Source: CAD feature listing. Evaluate the final solid. Frame: model axes, mm. A direction names the side the tool comes from. Give positions to 0.01 mm unless a question says otherwise; leave off trailing zeros. Write each loop counter-clockwise with the first axis right and the second up, starting at its lowest first coordinate (ties: lowest second). Pieces come first, ordered by that corner, then holes. Notation, with made-up numbers: (68, -11.75) -> (112, -11.75) arc R20 cw to (112, 15.25) -> close; hole circle Ø4 at (-7, 63). An arc over 180 degrees is marked (long way). Write item = value, one per line.
from build123d import *

# Parameters (mm, degrees)
F0_W     = 6.35
F0_H     = 2.54
F1_DEPTH = 19.05
F2_W     = 6.35
F2_H     = 5.588
F3_DEPTH = 2.54
F4_R     = 1.5875
F5_DEPTH = 25.4


with BuildPart() as f1:
    # F0 (on Top) → F1 (new body)
    with BuildSketch(Plane.XY):
        with Locations((15.875, 6.858)):
            Rectangle(F0_W, F0_H)
        Polygon((10.16, 2.54), (12.7, 2.54), (12.7, 5.588), (12.7, 8.128), (10.16, 8.128), align=None)
        Polygon((0, 2.54), (0, 0), (12.7, 0), (12.7, 2.54), (10.16, 2.54), align=None)
    extrude(amount=F1_DEPTH)

    # F2 (on face) → F3 (join)
    with BuildSketch(Plane(origin=(0, 0, 0), x_dir=(1, 0, 0), z_dir=(0, 0, -1))):
        with Locations((15.875, -2.794)):
            Rectangle(F2_W, F2_H)
    extrude(amount=-F3_DEPTH)

    # F4 (on face) → F5 (cut)
    with BuildSketch(Plane(origin=(0, 2.54, 0), x_dir=(-1, 0, 0), z_dir=(0, 1, 0))):
        with Locations((-5.08, 5.08)):
            Circle(F4_R)
    extrude(amount=-F5_DEPTH, mode=Mode.SUBTRACT)


solid = f1.part
(1) First-contact query: pin 1 (1.5 mm diameter, centred on x = 3, y = 1.5, fed in from -Z); pin 2 (7 mm diameter, centred on x = 17, z = 12.5, fed in from -Y); pin 3 (3 mm diameter, centred on x = 15, y = 3, fed in from +Z); pin 4 (2.5 mm diameter, centred on x = 5.08, z = 5.08, fed in from +Y). Flat tips, straight axial feed; report the tip coordinate or a pass-through.
Values follow:
pin_1 = 0
pin_2 = 5.59
pin_3 = 2.54
pin_4 = through
(2) Material intervals for line 1 (Z direction, x = 5.08, y = 1.35); line 2 (Y direction, x = 12.75, z = 14.5); line 3 (Y direction, x = 9, z = 13.75), sorted ascending.
Values follow:
line_1 = 0 to 3.49, 6.67 to 19.05
line_2 = 5.59 to 8.13
line_3 = 0 to 2.54
(3) Section query A-A (x = 5.08). Return loops of the section in (y, z), plus the area to 3 significant figures.
Values follow:
outline = (0, 0) -> (2.54, 0) -> (2.54, 3.49) -> (0, 3.49) -> close; (0, 6.67) -> (2.54, 6.67) -> (2.54, 19.05) -> (0, 19.05) -> close
area = 40.3 mm2
(4) Pull-direction query (X, two-part tool) for faces 4 (the face through (3.566, 1.288, 5.557)), 5 (the face through (16, 5.588, 11)), 6 (the face through (10.16, 5, 9)), 7 (the face through (19.05, 6, 7)); classes: pulls with the +X half, pulls with the -X half, needs draft (parallel to the pull), parting line crosses it, or undercut.
Values follow:
face_4 = undercut
face_5 = needs draft
face_6 = pulls with the -X half
face_7 = pulls with the +X half
(5) Section query B-B (z = 5.08). Return loops of the section in (x, y).
Values follow:
outline = (0, 0) -> (3.49, 0) -> (3.49, 2.54) -> (0, 2.54) -> close; (6.67, 0) -> (12.7, 0) -> (12.7, 5.59) -> (19.05, 5.59) -> (19.05, 8.13) -> (10.16, 8.13) -> (10.16, 2.54) -> (6.67, 2.54) -> close
(6) Access query for faces 1 (the face through (5, 2.54, 9)), 2 (the face through (9, 2, 19.05)), 3 (the face through (16, 3, 2.54)). Directions: +Z, -Z, +X, -X, +Y, -Y. A direction counts if a zero-diameter tool reaches every point of the face in a straight line with its end or side. Return the directions, or none.
Values follow:
face_1 = +Z, -Z, -X, +Y
face_2 = +Z, +X, -X, +Y, -Y
face_3 = +Z, +X, -Y
(7) Section query D-D (x = 16.25). Return loops of the section in (y, z).
Values follow:
outline = (0, 0) -> (8.13, 0) -> (8.13, 19.05) -> (5.59, 19.05) -> (5.59, 2.54) -> (0, 2.54) -> close
